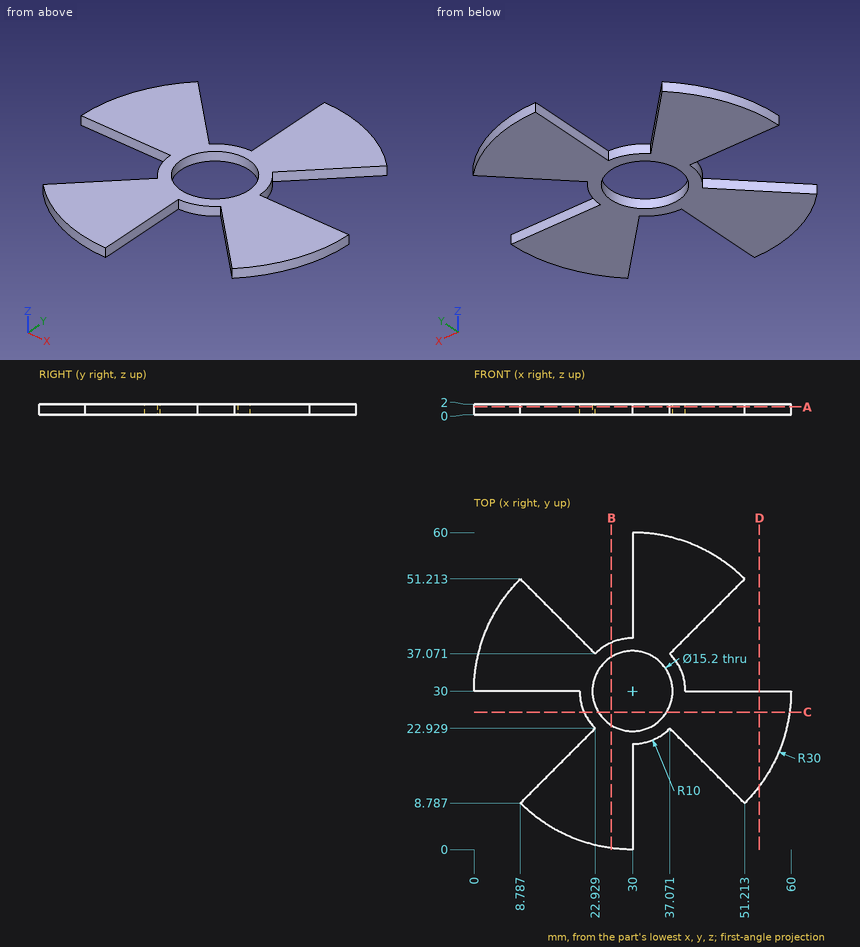
Design review of the part shown in the three views and the two pictorial views. Dimensions are in mm from the part's minimum x, y and z. Round coordinates to 2 decimals unless told otherwise and drop trailing zeros. Loops run counter-clockwise (first coordinate to the right, second up) from the corner with the lowest first, then second, coordinate; pieces in that order, holes last. Notation, with made-up numbers: (69.25, 57.5) - (116.25, 57.5) arc R21 ccw to (116.25, 92.5) - close; hole circle Ø5 at (31.5, 85.25). An arc over 180 degrees is marked (long way). Use CSV: the item, a comma, the result in double quotes.
(1) For line 1 (Y direction, x = 36, z = 0.7) (1 decimal); line 2 (X direction, y = 28.5, z = 0.45); line 3 (X direction, y = 49, z = 1.2), list the stretches that pass through material, from the lowest coordinate up.
Working result:
line 1,"y = 22 to 25.3, 34.7 to 59.4"
line 2,"x = 20.11 to 22.55, 37.45 to 59.96"
line 3,"x = 6.78 to 11, 30 to 49"
(2) Take a section at C-C, the plane y = 26. Give the boundary of the cut face in (x, z) (1 decimal).
Working result:
outline,"(20.8, 0) - (23.5, 0) - (23.5, 2) - (20.8, 2) - close; (36.5, 0) - (59.7, 0) - (59.7, 2) - (36.5, 2) - close"
(3) Take a section at B-B, the plane x = 26. Give the boundary of the cut face in (y, z) (1 decimal).
Working result:
outline,"(0.3, 0) - (23.5, 0) - (23.5, 2) - (0.3, 2) - close; (36.5, 0) - (39.2, 0) - (39.2, 2) - (36.5, 2) - close"
(4) Take a section at D-D, the plane x = 54. Give the boundary of the cut face in (y, z), plus the area to 3 significant figures.
Working result:
outline,"(12, 0) - (30, 0) - (30, 2) - (12, 2) - close"
area,"36.0 mm^2"
(5) Take a section at A-A, the plane z = 1.45. Give the boundary of the cut face in (x, y), plus the area to 3 significant figures.
Working result:
outline,"(0, 30) - (20, 30) arc R10 ccw to (22.93, 22.93) - (8.79, 8.79) arc R30 ccw to (30, 0) - (30, 20) arc R10 ccw to (37.07, 22.93) - (51.21, 8.79) arc R30 ccw to (60, 30) - (40, 30) arc R10 ccw to (37.07, 37.07) - (51.21, 51.21) arc R30 ccw to (30, 60) - (30, 40) arc R10 ccw to (22.93, 37.07) - (8.79, 51.21) arc R30 ccw to start; hole circle Ø15.2 at (30, 30)"
area,"1,390 mm^2"
(6) Clearance check with flat-ended pins moving along their axes: P1, Ø0.6, axis at x = 8, z = 1, coming from the -Y side; P2, Ø0.6, axis at y = 8, z = 0.5, coming from the +X side; P3, Ø1, axis at x = 53.5, z = 1, coming from the +Y side. State where each tip first meets the part, or that it passes through.
Working result:
P1,"stops at y = 30"
P2,"stops at x = 30"
P3,"stops at y = 30"
